from build123d import *

# Parameters (mm, degrees)
SKETCH_1_R      = 6.6
EXTRUDE_1_DEPTH = 3
FILLET_1_R      = 20


with BuildPart() as part:
    # Эскиз1 → Бобышка-Вытянуть1 (new body)
    with BuildSketch(Plane.XY):
        Polygon((152, 0), (-152, 0), (-152, 125), (-212, 125), (-212, -45), (212, -45), (212, 125), (152, 125), align=None)
        with Locations((-182, 95)):
            Circle(SKETCH_1_R, mode=Mode.SUBTRACT)
        with Locations((-182, 35)):
            Circle(SKETCH_1_R, mode=Mode.SUBTRACT)
        with Locations(Location((182, 35, 0), (0, 0, 180))):
            Circle(SKETCH_1_R, mode=Mode.SUBTRACT)
        with Locations(Location((182, 95, 0), (0, 0, 180))):
            Circle(SKETCH_1_R, mode=Mode.SUBTRACT)
    extrude(amount=EXTRUDE_1_DEPTH)

    # Скругление1
    fillet_1_edges = [part.edges().sort_by_distance(p)[0] for p in [
        (-152, 125, 1.5),
        (152, 125, 1.5),
    ]]
    fillet(fillet_1_edges, radius=FILLET_1_R)


solid = part.part
Input: part model. Units: mm. Frame: model coordinates. A direction names the side the tool comes from. Give positions to 0.01 mm unless a question says otherwise; leave off trailing zeros. Order: outer loops, then holes, each group sorted by start corner. A loop starts at its lowest first (then second) coordinate and runs counter-clockwise, first axis right, second up. Notation, with made-up numbers: (65.5, -19.75) - (114.5, -19.75) arc R20 cw to (114.5, 9.25) - close; hole circle Ø4 at (70.25, 9). An arc over 180 degrees is marked (long way). Write each question's results on one line, items separated by ' | '.
Item 1: Contact query for a flat-ended pin moving along its axis: pin 1 Ø17 at (x, y) = (182, 35) entering from +Z. Output: stop coordinate, or through.
A:
pin 1: stops at z = 3
Item 2: Section C-C (z = 0.8). Return loops of the section in (x, y), and give its area (3 significant figures).
A:
outline: (-212, -45) - (212, -45) - (212, 125) - (172, 125) arc R20 ccw to (152, 105) - (152, 0) - (-152, 0) - (-152, 105) arc R20 ccw to (-172, 125) - (-212, 125) - close; hole circle Ø13.2 at (-182, 35); hole circle Ø13.2 at (-182, 95); hole circle Ø13.2 at (182, 35); hole circle Ø13.2 at (182, 95) | area: 33,400 mm^2
Item 3: Section A-A (x = 182). Return loops of the section in (y, z).
A:
outline: (-45, 0) - (28.4, 0) - (28.4, 3) - (-45, 3) - close; (41.6, 0) - (88.4, 0) - (88.4, 3) - (41.6, 3) - close; (101.6, 0) - (125, 0) - (125, 3) - (101.6, 3) - close
Item 4: Access query for faces 1 (the cylindrical face through (-157.703, 118.986, 1.521)), 2 (the cylindrical face through (186.864, 90.539, 1.479)). Directions: +Z, -Z, +X, -X, +Y, -Y. A direction counts if a zero-diameter tool reaches every point of the face in a straight line with its end or side. Return the directions, or none.
A:
face 1: +Z, -Z, +Y | face 2: +Z, -Z
Item 5: Section B-B (y = 95). Return loops of the section in (x, z).
A:
outline: (-212, 0) - (-188.6, 0) - (-188.6, 3) - (-212, 3) - close; (-175.4, 0) - (-152, 0) - (-152, 3) - (-175.4, 3) - close; (152, 0) - (175.4, 0) - (175.4, 3) - (152, 3) - close; (188.6, 0) - (212, 0) - (212, 3) - (188.6, 3) - close
Item 6: Section D-D (y = 57). Return loops of the section in (x, z).
A:
outline: (-212, 0) - (-152, 0) - (-152, 3) - (-212, 3) - close; (152, 0) - (212, 0) - (212, 3) - (152, 3) - close
Item 7: Draft query along Y for faces 3 (the cylindrical face through (-188.594, 35.29, 1.479)), 4 (the cylindrical face through (157.703, 118.986, 1.521)), 5 (the flat face through (-3, -15, 0)), 6 (the cylindrical face through (188.594, 34.71, 1.479)). Return one class per face: released by +Y, released by -Y, zero draft, split by the parting line, or undercut.
A:
face 3: undercut | face 4: released by +Y | face 5: zero draft | face 6: undercut
Item 8: Material intervals for line 1 along Y through (x, z) = (182, 1.85); line 2 along X through (y, z) = (34.5, 2.55); line 3 along X through (y, z) = (15, 0.6), sorted ascending.
A:
line 1: y = -45 to 28.4, 41.6 to 88.4, 101.6 to 125 | line 2: x = -212 to -188.58, -175.42 to -152, 152 to 175.42, 188.58 to 212 | line 3: x = -212 to -152, 152 to 212
